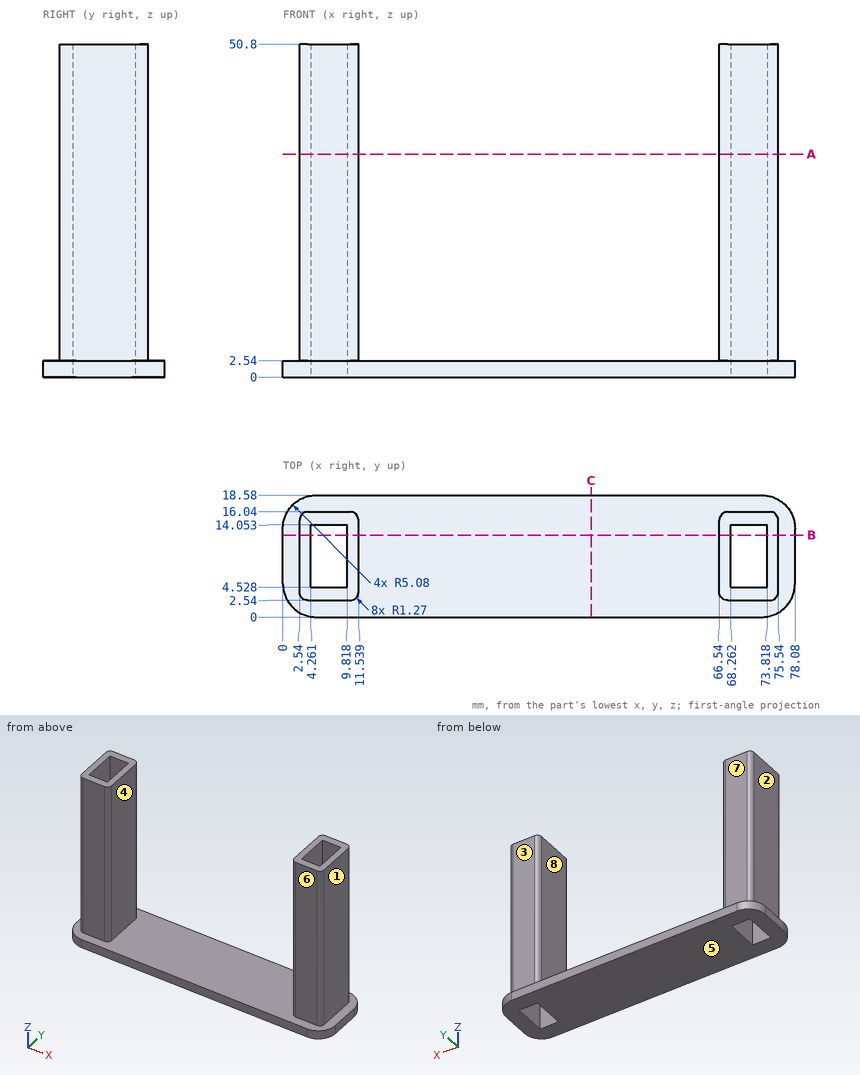
Can you work these out from the drawing? Everything is in mm from the part's minimum corner. A direction names the side the tool comes from. Coordinates: 2 decimals unless noted, no trailing zeros. Loops run counter-clockwise (first coordinate to the right, second up) from the corner with the lowest first, then second, coordinate; pieces in that order, holes last.
1) Imagine slicing it at A-A on z = 34. List the corners of the cut face in (x, y) for me.
2) Which directions (+Z, -Z, +X, -X, +Y, -Y) give clear straight access to the entire face, cutting with the end or side of a thin tool? Please do the marked faces 5, 6, 7 and 8.
3) Imagine slicing it at B-B on y = 12.5. List the corners of the cut face in (x, z) for me.
4) Thinking about a two-plate mould opening in X: for the marked faces 1, 2, 3 and 4, which applies, pulls with the +X half, pulls with the -X half, needs draft (parallel to the pull), parting line crosses it, or undercut?
5) Imagine slicing it at C-C on x = 47. List the corners of the cut face in (y, z) for me.
6) I need wall thicknesses on probe 1 along X at (y, z) = (7.5, 42.5); probe 2 along X at (y, z) = (4, 41); probe 3 along Y at (x, z) = (71.5, 39). Which ranges of each line are inside material? Lowest first, please.
7) For pin 1 (7 mm diameter, centred on x = 5.5, z = 27.5, fed in from -Y); pin 2 (5.5 mm diameter, centred on y = 8, z = 18, fed in from +X); pin 3 (2 mm diameter, centred on x = 38, y = 12.5, fed in from +Z), each with a flat end and sliding along its axis, tell me the tip position at first contact or that it passes through.
Completed:
1. outline: (2.54, 3.81) arc R1.27 ccw to (3.81, 2.54) - (10.27, 2.54) arc R1.27 ccw to (11.54, 3.81) - (11.54, 14.77) arc R1.27 ccw to (10.27, 16.04) - (3.81, 16.04) arc R1.27 ccw to (2.54, 14.77) - close; (66.54, 3.81) arc R1.27 ccw to (67.81, 2.54) - (74.27, 2.54) arc R1.27 ccw to (75.54, 3.81) - (75.54, 14.77) arc R1.27 ccw to (74.27, 16.04) - (67.81, 16.04) arc R1.27 ccw to (66.54, 14.77) - close; hole (4.26, 4.53) - (9.82, 4.53) - (9.82, 14.05) - (4.26, 14.05) - close; hole (68.26, 4.53) - (73.82, 4.53) - (73.82, 14.05) - (68.26, 14.05) - close
2. face 5: -Z, +X, -X, +Y, -Y
2. face 6: +Z, +X, -X, -Y
2. face 7: +Z, +X, -X, +Y
2. face 8: +Z, +Y, -Y
3. outline: (0, 0) - (4.26, 0) - (4.26, 50.8) - (2.54, 50.8) - (2.54, 2.54) - (0, 2.54) - close; (9.82, 0) - (68.26, 0) - (68.26, 50.8) - (66.54, 50.8) - (66.54, 2.54) - (11.54, 2.54) - (11.54, 50.8) - (9.82, 50.8) - close; (73.82, 0) - (78.08, 0) - (78.08, 2.54) - (75.54, 2.54) - (75.54, 50.8) - (73.82, 50.8) - close
4. face 1: pulls with the +X half
4. face 2: pulls with the -X half
4. face 3: needs draft
4. face 4: undercut
5. outline: (0, 0) - (18.58, 0) - (18.58, 2.54) - (0, 2.54) - close
6. probe 1: x = 2.54 to 4.26, 9.82 to 11.54, 66.54 to 68.26, 73.82 to 75.54
6. probe 2: x = 2.54 to 11.54, 66.54 to 75.54
6. probe 3: y = 2.54 to 4.53, 14.05 to 16.04
7. pin 1: stops at y = 2.54
7. pin 2: stops at x = 75.54
7. pin 3: stops at z = 2.54
